```python
from build123d import *

# Parameters (mm, degrees)
SKETCH1_W           = 206
SKETCH1_H           = 206
BOSS_EXTRUDE1_DEPTH = 303
FILLET1_R           = 10
SHELL1_T            = -3


with BuildPart() as part:
    # Sketch1 → Boss-Extrude1 (new body)
    with BuildSketch(Plane(origin=(0, 0, 0), x_dir=(1, 0, 0), z_dir=(0, 1, 0))):
        Rectangle(SKETCH1_W, SKETCH1_H)
    extrude(amount=BOSS_EXTRUDE1_DEPTH)

    # Fillet1
    fillet1_edges = [part.edges().sort_by_distance(p)[0] for p in [
        (103, 151.5, 103),
        (-103, 151.5, 103),
        (-103, 151.5, -103),
        (103, 151.5, -103),
    ]]
    fillet(fillet1_edges, radius=FILLET1_R)

    # Shell1
    shell1_openings = [part.faces().sort_by_distance(p)[0] for p in [
        (0, 303, 0),
    ]]
    offset(amount=SHELL1_T, openings=shell1_openings, kind=Kind.INTERSECTION)


solid = part.part
```
Geometry: final body of the model. Coordinates: model frame, mm. A direction names the side the tool comes from. Round coordinates to 2 decimals unless told otherwise and drop trailing zeros. Write each loop counter-clockwise with the first axis right and the second up, starting at its lowest first coordinate (ties: lowest second). Pieces come first, ordered by that corner, then holes. Notation, with made-up numbers: (37.5, 51.25) -> (43.5, 51.25) arc R19 cw to (43.5, 82.25) -> close; hole circle Ø2 at (16, -17.5). An arc over 180 degrees is marked (long way). Use CSV: the item, a comma, the result in double quotes. Start each with the question number.
Q1. Section B-B (x = 10.5). Return loops of the section in (y, z), plus the area to 3 significant figures.
Q2. Section C-C (z = -6.5). Return loops of the section in (x, y), plus the area to 3 significant figures.
Q3. Reachability of faces 1 (the face through (-98, 155.1, 97.9)), 2 (the face through (-103, 149, 1)) from +Z, -Z, +X, -X, +Y, -Y: full face, straight path, thin tool, end or side. Return the list, or none.
Q4. First-contact query: pin 1 Ø6 at (x, z) = (-10, 57) entering from +Y. Flat tip, straight axial feed; report the tip coordinate or a pass-through.
Q5. Line query: L1, parallel to Z at x = 37, y = 284; L2, parallel to Y at x = 49.5, z = -50. Output: solid intervals per line, ascending.
Q6. Pull-direction query (X, two-part tool) for faces 3 (the face through (-100.15, 153.62, 99.99)), 4 (the face through (-1, 0, -1)), 5 (the face through (100, 151, 1)); classes: pulls with the +X half, pulls with the -X half, needs draft (parallel to the pull), parting line crosses it, or undercut.
Q7. Section A-A (y = 226.5). Return loops of the section in (x, z).
Result sheet:
1,outline,"(0, -103) -> (303, -103) -> (303, -100) -> (3, -100) -> (3, 100) -> (303, 100) -> (303, 103) -> (0, 103) -> close"
1,area,"2,420 mm²"
2,outline,"(-103, 0) -> (103, 0) -> (103, 303) -> (100, 303) -> (100, 3) -> (-100, 3) -> (-100, 303) -> (-103, 303) -> close"
2,area,"2,420 mm²"
3,face 1,"+Y"
3,face 2,"+Z, -Z, -X, +Y, -Y"
4,pin 1,"y = 3"
5,L1,"-103 to -100, 100 to 103"
5,L2,"0 to 3"
6,face 3,"pulls with the -X half"
6,face 4,"needs draft"
6,face 5,"undercut"
7,outline,"(-103, -93) arc R10 ccw to (-93, -103) -> (93, -103) arc R10 ccw to (103, -93) -> (103, 93) arc R10 ccw to (93, 103) -> (-93, 103) arc R10 ccw to (-103, 93) -> close; hole (-100, -93) arc R7 ccw to (-93, -100) -> (93, -100) arc R7 ccw to (100, -93) -> (100, 93) arc R7 ccw to (93, 100) -> (-93, 100) arc R7 ccw to (-100, 93) -> close"
